Part model, mm, in its own coordinate system. Coordinates: 2 decimals unless noted, no trailing zeros. Write each loop counter-clockwise with the first axis right and the second up, starting at its lowest first coordinate (ties: lowest second). Pieces come first, ordered by that corner, then holes. Notation, with made-up numbers: (21.25, 58.25) - (46.25, 58.25) arc R22 ccw to (46.25, 72.25) - close; hole circle Ø8 at (62.5, 34.5). An arc over 180 degrees is marked (long way). Write each question's results on one line, items separated by ' | '.
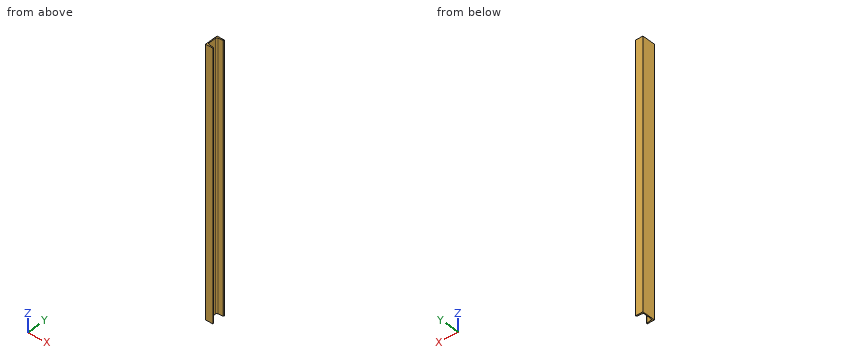
Autodesk Inventor part; units mm, degrees
ref_plane "Начальная плоскость" through (0, 0, 40) normal (0, 0, 1) x (1, 0, 0)
ref_plane "Конечная плоскость" through (0, 0, 1680) normal (0, 0, 1) x (1, 0, 0)
ref_plane "РабПлоскость4" through (-1.43, 1750, 40) normal (0, 0, -1) x (-1, 0, 0)
ref_plane "Начальная плоскость" through (0, 0, 40) normal (0, 0, 1) x (1, 0, 0)
ref_plane "Конечная плоскость" through (0, 0, 1680) normal (0, 0, 1) x (1, 0, 0)
sketch "Эскиз" plane through (0, 0, 0) normal (0, 0, 1) x (1, 0, 0)
  line L0 (-1.43, 0) -> (-1.43, 40)
  line L1 (-1.43, 40) -> (43.57, 40)
  line L2 (43.57, 40) -> (43.57, 38.1774)
  line L3 (39.9881, 34.1993) -> (11.2338, 31.1771)
  line L4 (4.07, 23.221) -> (4.07, 0)
  line L5 (4.07, 0) -> (-1.43, 0) construction
  line L6 (23.82, 40) -> (23.82, 32.5) construction
  line L7 (43.57, 34.5758) -> (43.57, 32.5) construction
  line L8 (43.57, 32.5) -> (23.82, 32.5) construction
  line L9 (0, 15) -> (0, -27) construction
  line L10 (-5.539, 0) -> (16.0067, 0) construction
  line L11 (-1.43, 0) -> (-1.43, -40)
  line L12 (-1.43, -40) -> (43.57, -40)
  line L13 (43.57, -40) -> (43.57, -38.1774)
  line L14 (39.9881, -34.1993) -> (11.2338, -31.1771)
  line L15 (4.07, -23.221) -> (4.07, 0)
  arc A0 (11.2338, 31.1771) -> (4.07, 23.221) centre (12.07, 23.221) ccw
  arc A1 (4.07, -23.221) -> (11.2338, -31.1771) centre (12.07, -23.221) ccw
  arc A2 (39.9881, 34.1993) -> (43.57, 38.1774) centre (39.57, 38.1774) ccw
  arc A3 (43.57, -38.1774) -> (39.9881, -34.1993) centre (39.57, -38.1774) ccw
  line L16 (0, 56) -> (0, -56) construction
  line L17 (-15.5135, 0) -> (54.308, 0) construction
  point P0 (4.07, 30.4242)
  point P1 (43.57, -34.5758)
  point P2 (4.07, -30.4242)
  point P3 (23.82, -40)
  point P4 (23.82, -32.5)
  dimension "d0" = 5.5
  dimension "d1" = 40
  dimension "d2" = 45
  dimension "d3" = 7.5
  dimension "d4" = 19.75
  dimension "d5" = 2.0758
  dimension "d23" = 8
  dimension "d24" = 4
  dimension "d25" = 1.43
extrude "Тело" add sketch "Эскиз" along normal up to surface (1640 mm away) from surface at 40
sketch "Sketch3" plane through (0, 0, 0) normal (0, 0, 1) x (1, 0, 0)
  line L0 (0, 0) -> (10, 0)
ref_plane "Work Plane3" through (0, 0, 0) normal (0, -1, 0) x (1, 0, 0)
sketch "Sketch4" plane through (0, 0, 0) normal (0, -1, 0) x (1, 0, 0)
  line L0 (-2, 40) -> (12, 40)
  line L1 (-2, 1680) -> (12, 1680)
  dimension "d29" = 1640
ref_plane "РабПлоскость4" through (-1.43, 1750, 40) normal (0, 0, -1) x (-1, 0, 0)
split "Разделение1" plane through (-1.43, 1750, 40) removes the side toward (0, 0, -1)
ref_plane "РабПлоскость5" through (-1.43, -1320, 1680) normal (0, 0, 1) x (1, 0, 0)
split "Разделение2" plane through (-1.43, -1320, 1680) removes the side toward (0, 0, 1)
equation "\"d0\" = G_T"
equation "\"d1\" = 0.5 * G_H"
equation "\"d2\" = G_W"
equation "\"d3\" = G_T1"
equation "\"d4\" = G_C"
equation "\"d23\" = G_IR"
equation "\"d24\" = G_ER"
equation "\"d25\" = ex"
equation "\"d6\" = G_L"
equation "\"G_W\" = 45"
equation "\"G_T\" = 5.5"
equation "\"G_T1\" = 7.5"
equation "\"G_NG\" = 0.105104"
equation "\"G_ER\" = 4"
equation "\"G_IR\" = 8"
equation "\"G_C\" = 19.75"
equation "\"G_L\" = d29"
equation "\"ex\" = 1.43"
properties part number "ISO 657/11 - CH 80 x 8 - 1640" material "Сталь, мягкая"
(1) Wall check: line 1 (Y direction, x = 39, z = 279.5); line 2 (X direction, y = -2, z = 1073); line 3 (Y direction, x = 41, z = 337). Give the ranges that are in metal, low to high. Write a range as from..to.
Return value:
line 1: y = -40..-34.1, 34.1..40 | line 2: x = -1.43..4.07 | line 3: y = -40..-34.44, 34.44..40
(2) Saw through at A-A on x = 27.5. Write the cut outline in (y, z), then the cut area to 3 significant figures.
Return value:
outline: (-40, 40) - (-32.89, 40) - (-32.89, 1680) - (-40, 1680) - close; (32.89, 40) - (40, 40) - (40, 1680) - (32.89, 1680) - close | area: 23,300 mm^2
(3) Saw through at C-C on y = 3.5. Write the cut outline in (x, z), then the cut area to 3 significant figures.
Return value:
outline: (-1.43, 40) - (4.07, 40) - (4.07, 1680) - (-1.43, 1680) - close | area: 9,020 mm^2
(4) Flat gauge pin, fed straight in: P1, Ø6, axis at y = 21.5, z = 1071, coming from the +X side. Where does the tip first touch, or does it go through?
Return value:
P1: stops at x = 4.17
(5) Saw through at B-B on z = 217.5. Write the cut outline in (x, y).
Return value:
outline: (-1.43, -40) - (43.57, -40) - (43.57, -38.18) arc R4 ccw to (39.99, -34.2) - (11.23, -31.18) arc R8 cw to (4.07, -23.22) - (4.07, 23.22) arc R8 cw to (11.23, 31.18) - (39.99, 34.2) arc R4 ccw to (43.57, 38.18) - (43.57, 40) - (-1.43, 40) - close
